```python
from build123d import *

# Parameters (mm, degrees)
BOSS_EXTRUDE1_START     = -20.6248
BOSS_EXTRUDE1_OUTLINE_W = 47.625
BOSS_EXTRUDE1_OUTLINE_H = 20.6248
BOSS_EXTRUDE1_DEPTH     = 25.4
BOSS_EXTRUDE1_2_DEPTH   = 4.7752
BOSS_EXTRUDE1_START_2   = 4.7752
BOSS_EXTRUDE1_3_DEPTH   = 20.6248
BOSS_EXTRUDE1_START_3   = -23.8125
BOSS_EXTRUDE1_4_DEPTH   = 47.625
SKETCH2_W               = 47.625
SKETCH2_H               = 25.4
BOSS_EXTRUDE2_DEPTH     = 4.7752
FILLET1_R               = 4.7752
SKETCH4_R               = 4.7625
CUT_EXTRUDE1_DEPTH      = 41.466993109
SKETCH5_R               = 4.7625
CUT_EXTRUDE2_DEPTH      = 41.466993109


with BuildPart() as part:
    # Boss-Extrude1: read off the stored shape, not the designer's step
    # Boss-Extrude1 outline → Boss-Extrude1 (new body)
    with BuildSketch(Plane.XZ.offset(-4.7752).offset(BOSS_EXTRUDE1_START)):
        with Locations((0, 15.0876)):
            Rectangle(BOSS_EXTRUDE1_OUTLINE_W, BOSS_EXTRUDE1_OUTLINE_H)
        with BuildLine():
            ThreePointArc((-18.972513521, 11.711023698), (-12.7, 19.05), (-6.427486479, 11.711023698))
            ThreePointArc((-6.427486479, 11.711023698), (-12.7, 6.35), (-18.972513521, 11.711023698))
        make_face(mode=Mode.SUBTRACT)
        with BuildLine():
            ThreePointArc((6.427486479, 11.711023698), (12.7, 19.05), (18.972513521, 11.711023698))
            ThreePointArc((18.972513521, 11.711023698), (12.7, 6.35), (6.427486479, 11.711023698))
        make_face(mode=Mode.SUBTRACT)
    extrude(amount=BOSS_EXTRUDE1_DEPTH)

    # Boss-Extrude1 2 outline → Boss-Extrude1 2 (add)
    with BuildSketch(Plane.XZ.offset(-4.7752)):
        with BuildLine():
            ThreePointArc((-18.972513521, 11.711023698), (-12.7, 6.35), (-6.427486479, 11.711023698))
            ThreePointArc((-6.427486479, 11.711023698), (-12.7, 19.05), (-18.972513521, 11.711023698))
        make_face()
        with BuildLine():
            ThreePointArc((6.427486479, 11.711023698), (12.7, 6.35), (18.972513521, 11.711023698))
            ThreePointArc((18.972513521, 11.711023698), (12.7, 19.05), (6.427486479, 11.711023698))
        make_face()
    extrude(amount=BOSS_EXTRUDE1_2_DEPTH)

    # Boss-Extrude1 3 outline → Boss-Extrude1 3 (cut)
    with BuildSketch(Plane.XY.offset(BOSS_EXTRUDE1_START_2)):
        with BuildLine():
            ThreePointArc((18.972513521, 11.711023698), (12.7, 19.05), (6.427486479, 11.711023698))
            ThreePointArc((6.427486479, 11.711023698), (12.7, 6.35), (18.972513521, 11.711023698))
        make_face()
        with BuildLine():
            ThreePointArc((-6.427486479, 11.711023698), (-12.7, 19.05), (-18.972513521, 11.711023698))
            ThreePointArc((-18.972513521, 11.711023698), (-12.7, 6.35), (-6.427486479, 11.711023698))
        make_face()
    extrude(amount=BOSS_EXTRUDE1_3_DEPTH, mode=Mode.SUBTRACT)

    # Boss-Extrude1 4 outline → Boss-Extrude1 4 (cut)
    with BuildSketch(Plane.YZ.offset(BOSS_EXTRUDE1_START_3)):
        Polygon((25.4, 25.4), (4.7752, 25.4), (25.4, 4.7752), align=None)
        Polygon((4.7752, 4.7752), (18.646847397, 4.7752), (4.7752, 18.646847397), align=None)
    extrude(amount=BOSS_EXTRUDE1_4_DEPTH, mode=Mode.SUBTRACT)

    # Sketch2 → Boss-Extrude2 (add)
    with BuildSketch(Plane(origin=(0, 0, 4.7752), x_dir=(-1, 0, 0), z_dir=(0, 0, -1))):
        with Locations((0, 12.7)):
            Rectangle(SKETCH2_W, SKETCH2_H)
    extrude(amount=BOSS_EXTRUDE2_DEPTH)

    # Fillet1
    fillet1_edges = [part.edges().sort_by_distance(p)[0] for p in [
        (0, 25.4, 4.7752),
        (0, 4.7752, 25.4),
    ]]
    fillet(fillet1_edges, radius=FILLET1_R)

    # Sketch4 → Cut-Extrude1 (cut, through all)
    with BuildSketch(Plane.XY.offset(4.7752)):
        with Locations((-12.7, 11.71067)):
            Circle(SKETCH4_R)
        with Locations(Location((12.7, 11.71067, 0), (0, 0, 180))):
            Circle(SKETCH4_R)
    extrude(amount=-CUT_EXTRUDE1_DEPTH, mode=Mode.SUBTRACT)

    # Sketch5 → Cut-Extrude2 (cut, through all)
    with BuildSketch(Plane(origin=(0, 4.7752, 0), x_dir=(1, 0, 0), z_dir=(0, 1, 0))):
        with Locations(Location((-12.7, -11.71067, 0), (0, 0, 270))):
            Circle(SKETCH5_R)
        with Locations(Location((12.7, -11.71067, 0), (0, 0, 90))):
            Circle(SKETCH5_R)
    extrude(amount=-CUT_EXTRUDE2_DEPTH, mode=Mode.SUBTRACT)


solid = part.part
```
Design review of the part built by this model. Coordinates are the model's own, in mm. A direction names the side the tool comes from. Coordinates: 2 decimals unless noted, no trailing zeros. Loops run counter-clockwise (first coordinate to the right, second up) from the corner with the lowest first, then second, coordinate; pieces in that order, holes last. Notation, with made-up numbers: (-19, -28.75) - (1, -28.75) arc R22 ccw to (1, 6.25) - close; hole circle Ø5 at (83.5, 21). An arc over 180 degrees is marked (long way). Use CSV: the item, a comma, the result in double quotes. Start each with the question number.
1) For pin 1 Ø3 at (x, z) = (-17, 6) entering from -Y; pin 2 Ø3 at (x, y) = (-9.5, 9.5) entering from +Z; pin 3 Ø4.5 at (x, y) = (-4, 13) entering from +Z; pin 4 Ø7.5 at (x, z) = (-12.7, 11.71) entering from +Y, all flat-tipped, find the tip position at first contact; note any pin that passes through.
2) Tool access review of faces 4 (the cylindrical face through (13.56, 18.99, 6.08)), 5 (the cylindrical face through (11.84, 6.11, 18.99)), 6 (the cylindrical face through (7.978, 2.421, 12.331)): name each direction out of +Z, -Z, +X, -X, +Y, -Y from which nothing blocks a thin tool from reaching the whole face with its end or side.
3) Wall thickness on L1, parallel to X at y = 13, z = 10.5; L2, parallel to Y at x = 12.7, z = 2.8; L3, parallel to X at y = 8.25, z = 17: over which ranges is each line inside the solid? List them lowest first. Write a range as from..to.
4) Consider section D-D on x = -2. Write out the cut boundary in (y, z).
5) Consider section A-A on x = 12.7. Write out the cut boundary in (y, z), then the cut area to 3 significant figures.
6) Consider section C-C on z = 10. Write out the cut boundary in (x, y).
7) The part is to be moulded in two halves that separate along X. For faces 1 (the cylindrical face through (0.333, 4.6, 25.046)), 2 (the flat face through (-23.812, 13, 13)), 3 (the cylindrical face through (8.157, 10.28, 2.421)), say which applies: +X half, -X half, draft (parallel to the pull), parting line (faces both ways), or undercut.
8) Consider section B-B on y = 9. Write out the cut boundary in (x, z).
Geometry says:
1,pin 1,"y = 0"
1,pin 2,"z = 4.78"
1,pin 3,"z = 19.43"
1,pin 4,"through"
2,face 4,"+Z"
2,face 5,"+Y"
2,face 6,"+Y, -Y"
3,L1,"-23.81..-19.04, -6.36..6.36, 19.04..23.81"
3,L2,"0..6.95, 16.47..25.4"
3,L3,"-23.81..-17.37, -8.03..8.03, 17.37..23.81"
4,outline,"(0, 0) - (25.4, 0) - (25.4, 2.8) arc R4.78 ccw to (24, 6.17) - (6.17, 24) arc R4.78 ccw to (2.8, 25.4) - (0, 25.4) - close; hole (4.78, 4.78) - (18.65, 4.78) - (4.78, 18.65) - close"
5,outline,"(0, 0) - (6.95, 0) - (6.95, 4.78) - (4.78, 4.78) - (4.78, 6.95) - (0, 6.95) - close; (0, 16.47) - (4.78, 16.47) - (4.78, 19.05) - (6.35, 19.05) - (6.35, 23.83) - (6.17, 24) arc R4.78 ccw to (2.8, 25.4) - (0, 25.4) - close; (16.47, 0) - (25.4, 0) - (25.4, 2.8) arc R4.78 ccw to (24, 6.17) - (23.83, 6.35) - (19.05, 6.35) - (19.05, 4.78) - (16.47, 4.78) - close"
5,area,"145 mm^2"
6,outline,"(-23.81, 0) - (-17.14, 0) - (-17.14, 4.78) - (-23.81, 4.78) - close; (-23.81, 13.42) - (-19.01, 13.42) arc R6.35 cw to (-18.45, 15.4) - (-18.45, 20.18) - (-23.81, 20.18) - close; (-8.26, 0) - (8.26, 0) - (8.26, 4.78) - (-8.26, 4.78) - close; (-6.95, 15.4) arc R6.35 cw to (-6.39, 13.42) - (6.39, 13.42) arc R6.35 cw to (6.95, 15.4) - (6.95, 20.18) - (-6.95, 20.18) - close; (17.14, 0) - (23.81, 0) - (23.81, 4.78) - (17.14, 4.78) - close; (18.45, 15.4) arc R6.35 cw to (19.01, 13.42) - (23.81, 13.42) - (23.81, 20.18) - (18.45, 20.18) - close"
7,face 1,"draft"
7,face 2,"-X half"
7,face 3,"undercut"
8,outline,"(-23.81, 0) - (-16.62, 0) - (-16.62, 4.78) - (-23.81, 4.78) - close; (-23.81, 14.42) - (-18.81, 14.42) arc R6.35 cw to (-17.86, 16.4) - (-17.86, 21.18) - (-23.81, 21.18) - close; (-8.78, 0) - (8.78, 0) - (8.78, 4.78) - (-8.78, 4.78) - close; (-7.54, 16.4) arc R6.35 cw to (-6.59, 14.42) - (6.59, 14.42) arc R6.35 cw to (7.54, 16.4) - (7.54, 21.18) - (-7.54, 21.18) - close; (16.62, 0) - (23.81, 0) - (23.81, 4.78) - (16.62, 4.78) - close; (17.86, 16.4) arc R6.35 cw to (18.81, 14.42) - (23.81, 14.42) - (23.81, 21.18) - (17.86, 21.18) - close"
